Drawing for the job (mm, zero at the part's lowest x, y, z). A direction names the side the tool comes from. Give positions to 0.01 mm unless a question says otherwise; leave off trailing zeros. Order: outer loops, then holes, each group sorted by start corner. A loop starts at its lowest first (then second) coordinate and runs counter-clockwise, first axis right, second up. Notation, with made-up numbers: M 12.25,7 L 18.25,7 A32 ccw 18.25,40 Z; hole C 74,29 d8. An arc over 180 degrees is marked long. Answer as a JSON object with one key per item and string values.
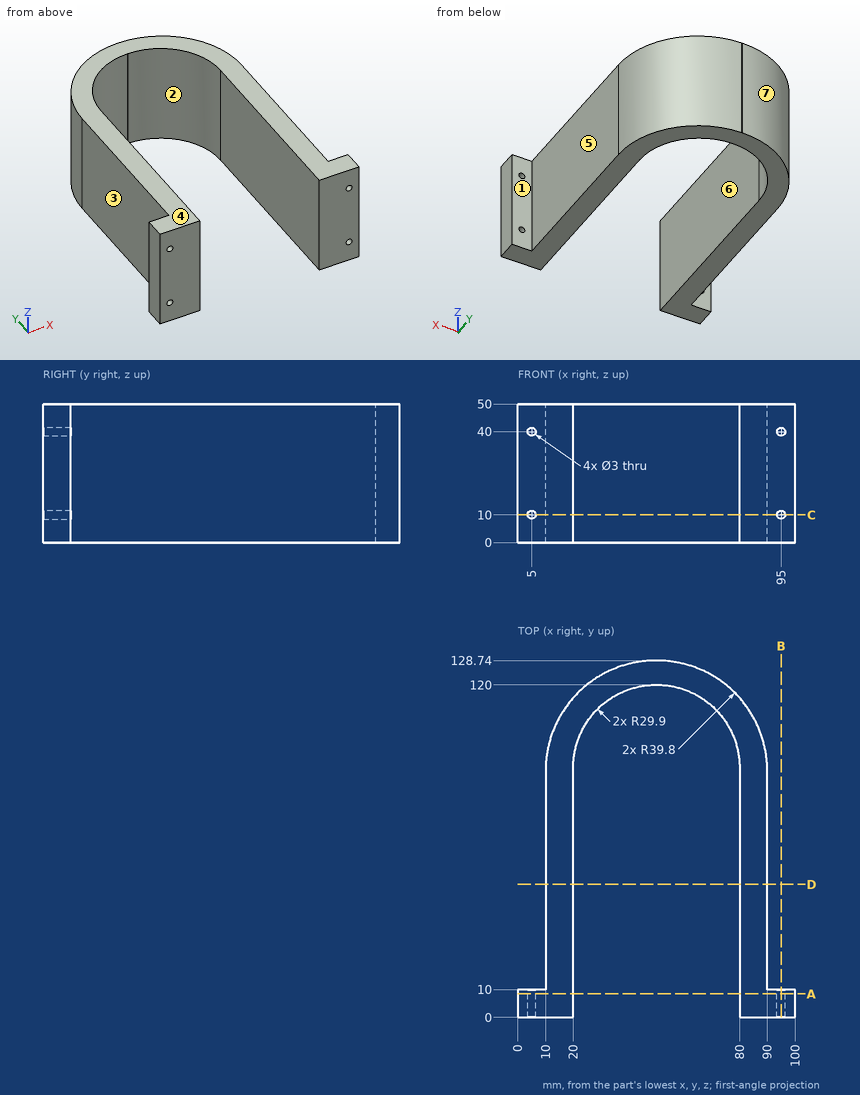
1. Cut at C-C on z = 10. Give the cut face in (x, y).
Worked answers:
{"outline": "M 0,0 L 3.5,0 L 3.5,10 L 0,10 Z; M 6.5,0 L 20,0 L 20,90.1 A29.9 cw 49.9,120 L 50.1,120 A29.9 cw 80,90.1 L 80,0 L 93.5,0 L 93.5,10 L 90,10 L 90,88.94 A39.8 ccw 50.2,128.74 L 49.8,128.74 A39.8 ccw 10,88.94 L 10,10 L 6.5,10 Z; M 96.5,0 L 100,0 L 100,10 L 96.5,10 Z"}
2. Probe line 1 along X through (y, z) = (2.75, 10); line 2 along Z through (x, y) = (95, 2); line 3 along X through (y, z) = (64, 3). List the from-to ranges inside material, lowest first.
Worked answers:
{"line 1": "x = 0 to 3.5, 6.5 to 20, 80 to 93.5, 96.5 to 100", "line 2": "z = 0 to 8.5, 11.5 to 38.5, 41.5 to 50", "line 3": "x = 10 to 20, 80 to 90"}
3. Cut at B-B on x = 95. Give the cut face in (y, z).
Worked answers:
{"outline": "M 0,0 L 10,0 L 10,8.5 L 0,8.5 Z; M 0,11.5 L 10,11.5 L 10,38.5 L 0,38.5 Z; M 0,41.5 L 10,41.5 L 10,50 L 0,50 Z"}
4. Cut at A-A on y = 8.5. Give the cut face in (x, z), plus the area to 3 significant figures.
Worked answers:
{"outline": "M 0,0 L 20,0 L 20,50 L 0,50 Z; M 80,0 L 100,0 L 100,50 L 80,50 Z; hole C 5,10 d3; hole C 5,40 d3; hole C 95,10 d3; hole C 95,40 d3", "area": "1,970 mm^2"}
5. Which spindle directions (+Z, -Z, +X, -X, +Y, -Y) get a long thin tool onto all of the face, cutting with end or side? Do the marked faces 1, 2, 3 and 4. Say none if no direction does.
Worked answers:
{"face 1": "+Z, -Z, +X, +Y", "face 2": "+Z, -Z, -Y", "face 3": "+Z, -Z, -X, +Y", "face 4": "+Z, +X, -X, +Y, -Y"}
6. Cut at D-D on y = 48. Give the cut face in (x, z), plus the area to 3 significant figures.
Worked answers:
{"outline": "M 10,0 L 20,0 L 20,50 L 10,50 Z; M 80,0 L 90,0 L 90,50 L 80,50 Z", "area": "1,000 mm^2"}
7. Two-plate mould, pull along X, no slides. Class the marked faces 5, 6 and 7: +X half, -X half, draft (parallel to the pull), parting line (faces both ways), or undercut.
Worked answers:
{"face 5": "+X half", "face 6": "undercut", "face 7": "-X half"}
8. Pin check, flat tips, straight feed: P1, Ø5, axis at x = 5, z = 35.5, coming from the +Y side; P2, Ø6, axis at y = 110, z = 36, coming from the +X side; P3, Ø2.5, axis at x = 5, z = 10, coming from the -Y side (3 decimals); P4, Ø25, axis at y = 47, z = 37, coming from the +X side. Stop position of each tip, or through.
Worked answers:
{"P1": "stops at y = 10", "P2": "stops at x = 85.67", "P3": "passes through", "P4": "stops at x = 90"}
